from build123d import *

# Parameters (mm, degrees)
SKETCH1_W           = 498.348
SKETCH1_H           = 165.1
BOSS_EXTRUDE1_DEPTH = 1.143
SKETCH2_W           = 69.85
SKETCH2_H           = 2.286
BOSS_EXTRUDE2_DEPTH = 3.175
LPATTERN1_COUNT     = 5
LPATTERN1_PITCH     = 98.8568
SKETCH3_W           = 96.5708
SKETCH3_H           = 16.239769195
SKETCH3_W_2         = 1.143
CUT_EXTRUDE1_DEPTH  = 264.517900145


with BuildPart() as part:
    # Sketch1 → Boss-Extrude1 (new, symmetric)
    with BuildSketch(Plane(origin=(0, 0, 0), x_dir=(1, 0, 0), z_dir=(0, 1, 0))):
        Rectangle(SKETCH1_W, SKETCH1_H)
    extrude(amount=BOSS_EXTRUDE1_DEPTH, both=True)

    # Sketch2 → Boss-Extrude2 (add)
    with BuildSketch(Plane(origin=(0, 0, -82.55), x_dir=(-1, 0, 0), z_dir=(0, 0, -1))):
        with Locations((-197.7136, 0)):
            Rectangle(SKETCH2_W, SKETCH2_H)
    boss_extrude2 = extrude(amount=BOSS_EXTRUDE2_DEPTH)

    # LPattern1: Boss-Extrude2 ×5
    with Locations(*[(-i * LPATTERN1_PITCH, 0, 0) for i in range(1, LPATTERN1_COUNT)]):
        add(boss_extrude2)

    # Sketch3 → Cut-Extrude1 (cut, through all)
    with BuildSketch(Plane.XZ.offset(1.143)):
        with Locations((-98.8568, 74.430115403)):
            Rectangle(SKETCH3_W, SKETCH3_H)
        with Locations((-48.8569, 74.430115403)):
            Rectangle(SKETCH3_W_2, SKETCH3_H)
        with Locations((-49.9999, 74.430115403)):
            Rectangle(SKETCH3_W_2, SKETCH3_H)
        with Locations((0, 74.430115403)):
            Rectangle(SKETCH3_W, SKETCH3_H)
    extrude(amount=-CUT_EXTRUDE1_DEPTH, mode=Mode.SUBTRACT)


solid = part.part
Design review of the part built by this model. Coordinates are the model's own, in mm. Coordinates: 2 decimals unless noted, no trailing zeros. Loops run counter-clockwise (first coordinate to the right, second up) from the corner with the lowest first, then second, coordinate; pieces in that order, holes last. Notation, with made-up numbers: M 27.5,40 L 60.5,40 A3 cw 60.5,44 Z; hole C -19.5,57.5 d3. An arc over 180 degrees is marked long. Use one line per item in the form item = value.
(1) For line 1 along Z through (x, y) = (-62.5, 0.55); line 2 along X through (y, z) = (0.8, 72.5); line 3 along Z through (x, y) = (6, 0) (3 decimals), list the stretches that pass through material, from the lowest coordinate up. Write a range as from..to.
Return value:
line_1 = -82.55..66.31
line_2 = -249.17..-147.14, 48.29..249.17
line_3 = -85.725..66.31
(2) Clearance check with flat-ended pins moving along their axes: P1, Ø1.1, axis at y = -0.5, z = -84, coming from the +X side; P2, Ø1.1, axis at y = -0.5, z = -84, coming from the -X side; P3, Ø1.1, axis at x = 237.5, y = 0, coming from the -Z side. State where each tip first meets the part, or that it passes through.
Return value:
P1 = 232.64
P2 = -232.64
P3 = -82.55
(3) Consider section A-A (y = -0.75). Write out the cut boundary in (x, z) (3 decimals), and give its area (3 significant figures).
Return value:
outline = M -249.174,-82.55 L -232.639,-82.55 L -232.639,-85.725 L -162.789,-85.725 L -162.789,-82.55 L -133.782,-82.55 L -133.782,-85.725 L -63.932,-85.725 L -63.932,-82.55 L -34.925,-82.55 L -34.925,-85.725 L 34.925,-85.725 L 34.925,-82.55 L 63.932,-82.55 L 63.932,-85.725 L 133.782,-85.725 L 133.782,-82.55 L 162.789,-82.55 L 162.789,-85.725 L 232.639,-85.725 L 232.639,-82.55 L 249.174,-82.55 L 249.174,82.55 L 48.285,82.55 L 48.285,66.31 L -147.142,66.31 L -147.142,82.55 L -249.174,82.55 Z
area = 80,200 mm2
(4) Consider section C-C (x = -102.5). Write out the cut boundary in (y, z) (3 decimals), and give its area (3 significant figures).
Return value:
outline = M -1.143,-85.725 L 1.143,-85.725 L 1.143,66.31 L -1.143,66.31 Z
area = 348 mm2
(5) Consider section B-B (x = 52.5). Write out the cut boundary in (y, z).
Return value:
outline = M -1.14,-82.55 L 1.14,-82.55 L 1.14,82.55 L -1.14,82.55 Z
